For this review, use the dimensioned drawing (mm, ordinates from the lowest corner) and the shaded views. A direction names the side the tool comes from. Round coordinates to 2 decimals unless told otherwise and drop trailing zeros. Write each loop counter-clockwise with the first axis right and the second up, starting at its lowest first coordinate (ties: lowest second). Pieces come first, ordered by that corner, then holes. Notation, with made-up numbers: M -27.75,81 L -11.75,81 A9 ccw -11.75,92 Z; hole C 41,-2.5 d3. An arc over 180 degrees is marked long. Use one line per item in the form item = value. Start each with the question number.
Item 1: For the marked faces 4 and 5, list the 3-axis set-ups (+Z, -Z, +X, -X, +Y, -Y) from which the entire face can be reached by the end or side of a thin tool; tool diameter is ignored.
Item 2: Add section C-C (x = 23). State the section outline as (y, z) points, and give its area (3 significant figures).
Item 3: Draft analysis for pull direction X (two halves, no side actions). For the marked faces 1, 2 and 3, state which applies: released by +X, released by -X, zero draft, split by the parting line, or undercut.
Item 4: Add section A-A (y = 4.9). State the section outline as (x, z) points.
Item 5: Add section B-B (z = 12.75). State the section outline as (x, y) points, and give its area (3 significant figures).
Item 6: For line 1 (X direction, y = 3.4, z = 14.75); line 2 (Z direction, x = 30.5, y = 1.9); line 3 (Y direction, x = 18.5, z = 5.75), list the stretches that pass through material, from the lowest coordinate up. Write a range as [from, to].
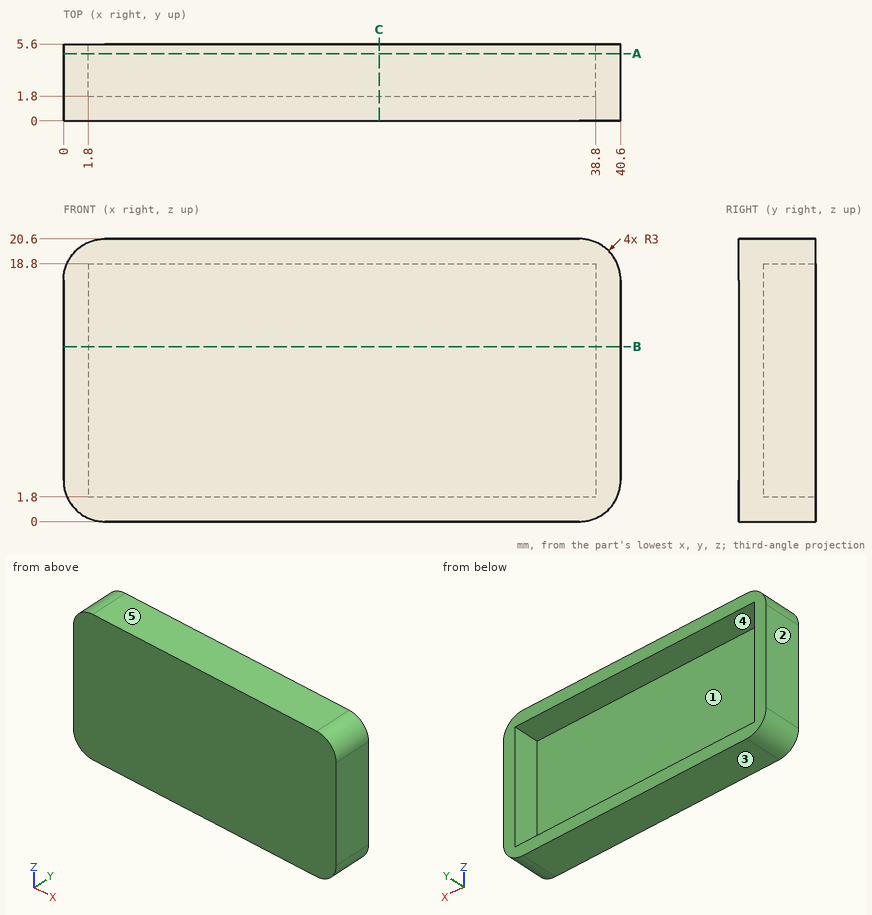
Calculated:
q1.face_4 = +Y
q1.face_5 = +Z, +X, -X, +Y, -Y
q2.outline = M 0,0 L 5.6,0 L 5.6,1.8 L 1.8,1.8 L 1.8,18.8 L 5.6,18.8 L 5.6,20.6 L 0,20.6 Z
q2.area = 50.8 mm^2
q3.face_1 = undercut
q3.face_2 = released by -X
q3.face_3 = zero draft
q4.outline = M 0,3 A3 ccw 3,0 L 37.6,0 A3 ccw 40.6,3 L 40.6,17.6 A3 ccw 37.6,20.6 L 3,20.6 A3 ccw 0,17.6 Z; hole M 1.8,1.8 L 38.8,1.8 L 38.8,18.8 L 1.8,18.8 Z
q5.outline = M 0,0 L 40.6,0 L 40.6,5.6 L 38.8,5.6 L 38.8,1.8 L 1.8,1.8 L 1.8,5.6 L 0,5.6 Z
q5.area = 86.8 mm^2
q6.line_1 = [0, 1.8], [38.8, 40.6]
q6.line_2 = [0, 1.8], [18.8, 20.6]
q6.line_3 = [0, 1.8]
